```python
from build123d import *

# Parameters (mm, degrees)
SKETCH1_R                     = 11
SKETCH1_R_2                   = 5
SKETCH1_R_3                   = 3.5
SKETCH1_R_4                   = 2
BODY_DEPTH                    = 36
SKETCH1_3_R                   = 5
SKETCH1_3_R_2                 = 3.5
COLLAR_1_DEPTH                = 1.35
SKETCH1_4_R                   = 3.5
SKETCH1_4_R_2                 = 2
COLLAR_2_DEPTH                = 3.15
CAP_START                     = -1.5
SKETCH4_R                     = 11
SKETCH4_R_2                   = 10.5
CAP_RING_DEPTH                = 0.001
SKETCH1_5_R                   = 2
SHAFT_DEPTH                   = 14.85
KEY_START                     = -9.3
KEY_WAY_DEPTH                 = 9.3
SKETCH2_R                     = 5
SKETCH2_R_2                   = 1.5
RECESS_FOR_MOTOR_COLLAR_DEPTH = 1
SKETCH2_2_R                   = 1.5
RECESS_FOR_MOTOR_SHAFT_DEPTH  = 10.3


with BuildPart() as part:
    # Sketch1 → Body (new body)
    # profile 1 of 4: a face of its own
    with BuildSketch(Plane.XY):
        Circle(SKETCH1_R)
        Circle(SKETCH1_R_2, mode=Mode.SUBTRACT)
    # profile 2 of 4: a face of its own
    with BuildSketch(Plane.XY):
        Circle(SKETCH1_R_2)
        Circle(SKETCH1_R_3, mode=Mode.SUBTRACT)
    # profile 3 of 4: a face of its own
    with BuildSketch(Plane.XY):
        Circle(SKETCH1_R_3)
        Circle(SKETCH1_R_4, mode=Mode.SUBTRACT)
    # profile 4 of 4: a face of its own
    with BuildSketch(Plane.XY):
        Circle(SKETCH1_R_4)
    extrude(amount=-BODY_DEPTH)

    # Sketch1_3 → Collar 1 (add)
    with BuildSketch(Plane.XY):
        with Locations(Location((0, 0, 0), (0, 0, 180))):
            Circle(SKETCH1_3_R)
        with Locations(Location((0, 0, 0), (0, 0, 180))):
            Circle(SKETCH1_3_R_2, mode=Mode.SUBTRACT)
    extrude(amount=COLLAR_1_DEPTH)

    # Sketch1_4 → Collar 2 (add)
    with BuildSketch(Plane.XY):
        Circle(SKETCH1_4_R)
        Circle(SKETCH1_4_R_2, mode=Mode.SUBTRACT)
    extrude(amount=COLLAR_2_DEPTH)

    # Sketch4 → Cap Ring (cut)
    with BuildSketch(Plane.XY.offset(CAP_START)):
        Circle(SKETCH4_R)
        Circle(SKETCH4_R_2, mode=Mode.SUBTRACT)
    extrude(amount=-CAP_RING_DEPTH, mode=Mode.SUBTRACT)

    # Sketch1_5 → Shaft (add)
    with BuildSketch(Plane.XY):
        Circle(SKETCH1_5_R)
    extrude(amount=SHAFT_DEPTH)

    # Sketch3 → Key Way (cut)
    with BuildSketch(Plane.XY.offset(14.85).offset(KEY_START)):
        with BuildLine():
            Line((-1.322875656, 1.5), (0, 1.5))
            Line((0, 1.5), (1.322875656, 1.5))
            ThreePointArc((1.322875656, 1.5), (0, 2), (-1.322875656, 1.5))
        make_face()
    extrude(amount=KEY_WAY_DEPTH, mode=Mode.SUBTRACT)

    # Sketch2 → Recess for Motor Collar (cut)
    with BuildSketch(Plane(origin=(0, 0, -36), x_dir=(-1, 0, 0), z_dir=(0, 0, -1))):
        Circle(SKETCH2_R)
        Circle(SKETCH2_R_2, mode=Mode.SUBTRACT)
    extrude(amount=-RECESS_FOR_MOTOR_COLLAR_DEPTH, mode=Mode.SUBTRACT)

    # Sketch2_2 → Recess for Motor Shaft (cut)
    with BuildSketch(Plane(origin=(0, 0, -36), x_dir=(-1, 0, 0), z_dir=(0, 0, -1))):
        Circle(SKETCH2_2_R)
    extrude(amount=-RECESS_FOR_MOTOR_SHAFT_DEPTH, mode=Mode.SUBTRACT)


solid = part.part
```
Could you check a few things on this model? Use its own coordinates, in mm. A direction names the side the tool comes from. Round coordinates to 2 decimals unless told otherwise and drop trailing zeros. Write each loop counter-clockwise with the first axis right and the second up, starting at its lowest first coordinate (ties: lowest second). Pieces come first, ordered by that corner, then holes. Notation, with made-up numbers: M -39.75,5.5 L -35.75,5.5 A6 cw -35.75,13.5 Z; hole C 89,-2.5 d8. An arc over 180 degrees is marked long. Answer in a Markdown table with one row per item. Add a question column.
Q1. Will these pins go through, and if not, where does the flat tip stop? pin 1 Ø1.5 at (x, z) = (3.5, 5) entering from -Y; pin 2 Ø3 at (x, z) = (8, -10.5) entering from +Y; pin 3 Ø8 at (x, y) = (-0.5, 0.5) entering from -Z; pin 4 Ø0.8 at (x, z) = (-0.5, 9.5) entering from +Y.
Q2. Imagine slicing it at C-C (z = -23.5). Please give me the cut outline in (x, y), then the cut area to 3 significant figures.
Q3. If I drill on line 1 (Y direction, x = 0, z = -35.4); line 2 (Z direction, x = 2, y = -1.5); line 3 (Z direction, x = -3.5, y = 6), over which ranges is the centre line in solid material (lowest first)? Write a range as from..to.
Q4. On a 3-axis mill with a long thin cutter (end or side, diameter ignored), from which of +Z, -Z, +X, -X, +Y, -Y can I reach the whole of each face in a straight line? I mean faces 1 (the flat face through (0, 1.5, 10)), 2 (the flat face through (2, -5, -36)), 3 (the cylindrical face through (-2.38, -10.74, -18.51)), 4 (the flat face through (1.2, 1.2, -35)), 5 (the cylindrical face through (3.233, -1.341, 2.237)). Say none if no direction works.
Values:
| question | item | result |
|---|---|---|
| 1 | pin 1 | through |
| 1 | pin 2 | y = 8.87 |
| 1 | pin 3 | z = -35 |
| 1 | pin 4 | y = 1.5 |
| 2 | outline | C 0,0 d22 |
| 2 | area | 380 mm^2 |
| 3 | line 1 | -11..-5, 5..11 |
| 3 | line 2 | -35..3.15 |
| 3 | line 3 | -36..0 |
| 4 | face 1 | +Z, +X, -X, +Y |
| 4 | face 2 | -Z, +X, -X, +Y, -Y |
| 4 | face 3 | +Z, -Z |
| 4 | face 4 | -Z |
| 4 | face 5 | +Z |
